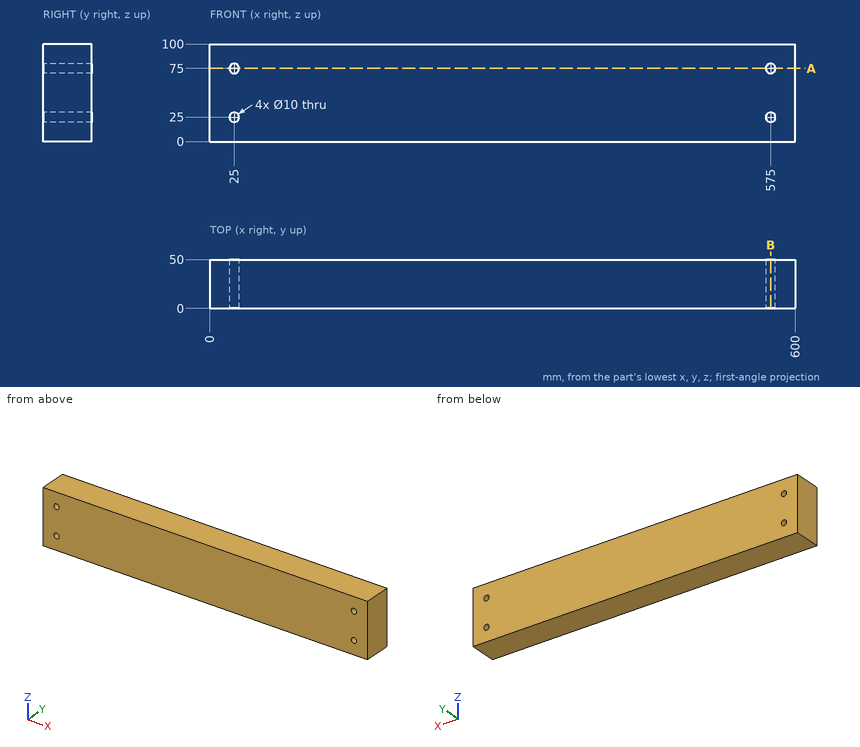
Design review of the part shown in the three views and the two pictorial views. Dimensions are in mm from the part's minimum x, y and z. Give positions to 0.01 mm unless a question says otherwise; leave off trailing zeros. Write each loop counter-clockwise with the first axis right and the second up, starting at its lowest first coordinate (ties: lowest second). Pieces come first, ordered by that corner, then holes. Notation, with made-up numbers: (58.25, -27) - (71.25, -27) arc R16 cw to (71.25, 4) - close; hole circle Ø9 at (-29.5, 35.25). An arc over 180 degrees is marked (long way). Return JSON: item names as keys, results as strings. Group by question number.
(1) Insertion check: pin 1 (16 mm diameter, centred on x = 575, z = 25, fed in from -Y). The pin has a flat end and moves straight along its axis. Give the tip position at first contact, or say it passes through.
(2) To check wall thickness, follow probe 1 along Z at (x, y) = (25, 39.5); probe 2 along X at (y, z) = (38.5, 27); probe 3 along X at (y, z) = (22, 27.5). State the ranges of each line that lie inside material, in increasing order.
(3) We need section A-A, the plane z = 75. Give the boundary of the cut face in (x, y).
(4) We need section B-B, the plane x = 575. Give the boundary of the cut face in (y, z), then the cut area to 3 significant figures.
Reported:
{
 "1": {"pin 1": "stops at y = 0"},
 "2": {"probe 1": "z = 0 to 20, 30 to 70, 80 to 100", "probe 2": "x = 0 to 20.42, 29.58 to 570.42, 579.58 to 600", "probe 3": "x = 0 to 20.67, 29.33 to 570.67, 579.33 to 600"},
 "3": {"outline": "(0, 0) - (20, 0) - (20, 50) - (0, 50) - close; (30, 0) - (570, 0) - (570, 50) - (30, 50) - close; (580, 0) - (600, 0) - (600, 50) - (580, 50) - close"},
 "4": {"outline": "(0, 0) - (50, 0) - (50, 20) - (0, 20) - close; (0, 30) - (50, 30) - (50, 70) - (0, 70) - close; (0, 80) - (50, 80) - (50, 100) - (0, 100) - close", "area": "4,000 mm2"}
}
